Read the model definition and answer for the solid it produces. Units are mm, in the model's axes. Give positions to 0.01 mm unless a question says otherwise; leave off trailing zeros. Loops run counter-clockwise (first coordinate to the right, second up) from the corner with the lowest first, then second, coordinate; pieces in that order, holes last.
(1) Determine the mould class of faces 1 (the face through (-21, 3, -12.967)), 2 (the face through (-24.19, 3.46, -5.01)), 3 (the face through (-19.2, 3.46, 5.19)) for opening direction X: pulls with the +X half, pulls with the -X half, needs draft (parallel to the pull), parting line crosses it, or undercut.
(2) Each of these flat-tipped pins is pushed along its axis until it touches: P1, Ø1.5, axis at y = 2.5, z = 1.5, coming from the +X side; P2, Ø1.5, axis at y = 1, z = 8, coming from the -X side; P3, Ø2, axis at y = 3, z = 1, coming from the -X side. Where does it stop, or does it pass through?
(3) Find section A-A, the plane y = 1.5. Write down the section's boundary in (x, z), then the cut area to 3 significant figures.
(4) Straight lines are drawn through the part: probe 1 along Z at (x, y) = (-21.25, 2); probe 2 along Z at (x, y) = (-18.5, 2.25); probe 3 along X at (y, z) = (4.25, 8.75). For each, find the intervals that lie inside material, in ascending order.
```python
from build123d import *

# Parameters (mm, degrees)
SKETCH1_R           = 2.5
BOSS_EXTRUDE1_DEPTH = 7
FILLET1_R           = 2
FILLET2_R           = 0.5


with BuildPart() as part:
    # Sketch1 → Boss-Extrude1 (new body)
    with BuildSketch(Plane(origin=(0, 0, 0), x_dir=(1, 0, 0), z_dir=(0, 1, 0))):
        Polygon((-23.791870344, 12.96668262), (-17.291870344, 12.96668262), (-16.541870344, -2.03331738), (-6.271908742, -7.297228373), (-6.271908742, -12.297228373), (-34.811831945, -12.297228373), (-34.811831945, -7.297228373), (-24.541870344, -2.03331738), align=None)
        with Locations((-20.541870344, -7.297228373)):
            Circle(SKETCH1_R, mode=Mode.SUBTRACT)
    extrude(amount=BOSS_EXTRUDE1_DEPTH)

    # Fillet1
    fillet1_edges = [part.edges().sort_by_distance(p)[0] for p in [
        (-23.791870344, 3.5, -12.96668262),
        (-17.291870344, 3.5, -12.96668262),
        (-16.541870344, 3.5, 2.03331738),
        (-6.271908742, 3.5, 7.297228373),
        (-34.811831945, 3.5, 7.297228373),
        (-24.541870344, 3.5, 2.03331738),
    ]]
    fillet(fillet1_edges, radius=FILLET1_R)

    # Fillet2
    fillet2_edges = [part.edges().sort_by_distance(p)[0] for p in [
        (-20.541870344, 0, 12.297228373),
        (-34.811831945, 7, 10.408378726),
        (-34.811831945, 0, 10.408378726),
        (-20.541870344, 7, 12.297228373),
        (-6.271908742, 3.5, 12.297228373),
        (-34.811831945, 3.5, 12.297228373),
        (-11.436968701, 0, 4.649855681),
        (-11.436968701, 7, 4.649855681),
        (-24.185541966, 0, -5.093250169),
        (-20.541870344, 0, -12.96668262),
        (-16.898198721, 0, -5.093250169),
        (-6.271908742, 0, 10.408378726),
        (-29.646771987, 0, 4.649855681),
        (-17.815918651, 0, -12.415777246),
        (-23.267822036, 0, -12.415777246),
        (-34.518365815, 0, 7.476580302),
        (-6.565374872, 0, 7.476580302),
        (-6.271908742, 7, 10.408378726),
        (-23.041870344, 7, 7.297228373),
        (-24.185541966, 7, -5.093250169),
        (-29.646771987, 7, 4.649855681),
        (-16.898198721, 7, -5.093250169),
        (-20.541870344, 7, -12.96668262),
        (-17.815918651, 7, -12.415777246),
        (-23.267822036, 7, -12.415777246),
        (-34.518365815, 7, 7.476580302),
        (-6.565374872, 7, 7.476580302),
        (-16.281980837, 0, 1.865429111),
        (-16.281980837, 7, 1.865429111),
        (-24.80175985, 0, 1.865429111),
        (-24.80175985, 7, 1.865429111),
        (-23.041870344, 0, 7.297228373),
    ]]
    fillet(fillet2_edges, radius=FILLET2_R)


solid = part.part
```
Entries:
1. face 1: needs draft
1. face 2: pulls with the -X half
1. face 3: undercut
2. P1: stops at x = -15.96
2. P2: stops at x = -34.81
2. P3: stops at x = -24.9
3. outline: (-34.81, 8.52) arc R2 ccw to (-33.72, 6.74) - (-25.57, 2.56) arc R2 cw to (-24.48, 0.88) - (-23.89, -11.07) arc R2 ccw to (-21.89, -12.97) - (-19.19, -12.97) arc R2 ccw to (-17.2, -11.07) - (-16.6, 0.88) arc R2 cw to (-15.51, 2.56) - (-7.36, 6.74) arc R2 ccw to (-6.27, 8.52) - (-6.27, 11.8) arc R0.5 ccw to (-6.77, 12.3) - (-34.31, 12.3) arc R0.5 ccw to (-34.81, 11.8) - close; hole circle Ø5 at (-20.54, 7.3)
3. area: 326 mm2
4. probe 1: z = -12.97 to 4.9, 9.69 to 12.3
4. probe 2: z = -12.84 to 5.85, 8.74 to 12.3
4. probe 3: x = -34.81 to -22.58, -18.51 to -6.27
